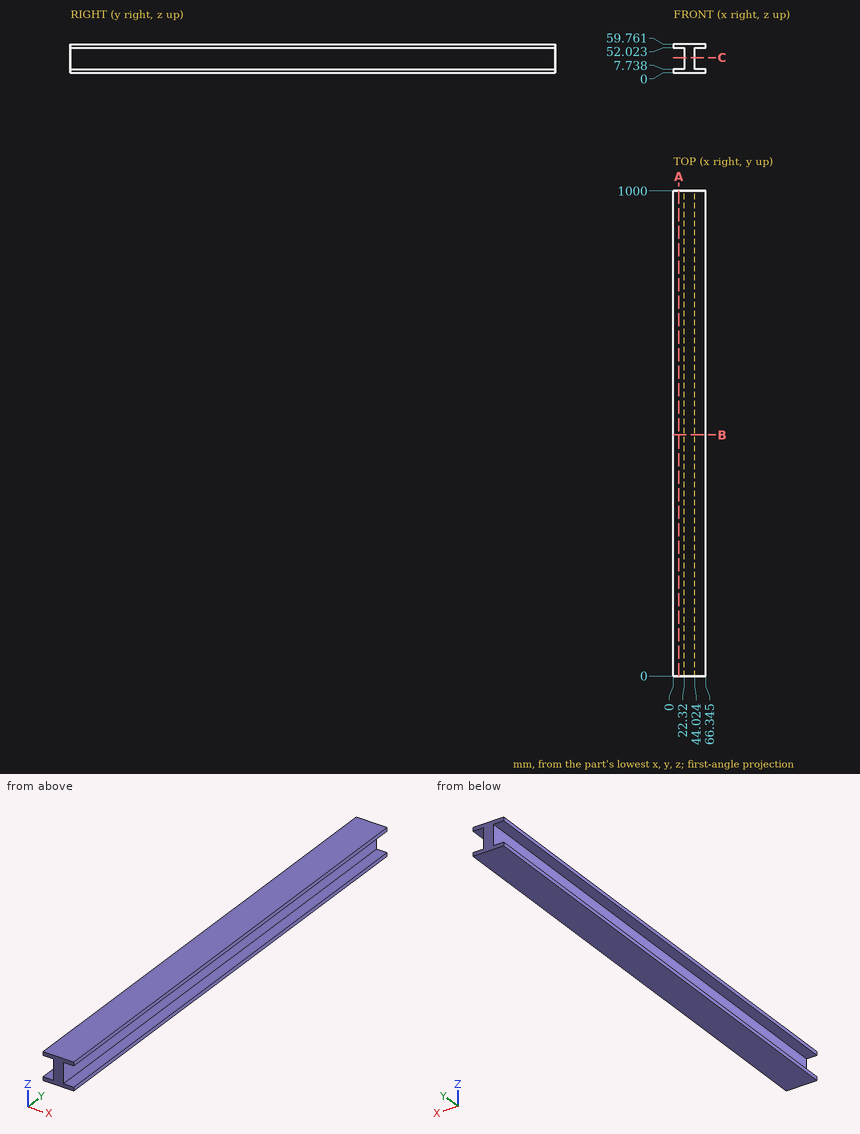
Geometry: see drawing. Coordinates: mm, zero at the bounding-box minimum. Round coordinates to 2 decimals unless told otherwise and drop trailing zeros. Loops run counter-clockwise (first coordinate to the right, second up) from the corner with the lowest first, then second, coordinate; pieces in that order, holes last. Notation, with made-up numbers: M 25,-21 L 75,-21 A5 ccw 75,-14 Z; hole C 79,88 d2. An arc over 180 degrees is marked long. Use a Markdown table: item, result. Add a question column.
1. Cut plane A-A, the plane x = 11.5. Output: boundary loops of the cut face in (y, z).
2. Contact query for flat-ended pins moving along their axis: pin 1 (8 mm diameter, centred on y = 384, z = 34, fed in from +X); pin 2 (8 mm diameter, centred on y = 864, z = 43, fed in from -X). Output: stop coordinate, or through.
3. Cut plane C-C, the plane z = 31.5. Output: boundary loops of the cut face in (x, y) (1 decimal).
4. Ray query, line 1 along Z through (x, y) = (46, 421); line 2 along X through (y, z) = (181.5, 21) (1 decimal). Return the intervals inside material, ascending. Write a range as [from, to].
5. Cut plane B-B, the plane y = 497. Output: boundary loops of the cut face in (x, z) (1 decimal).
Solution:
| question | item | result |
|---|---|---|
| 1 | outline | M 0,0 L 1000,0 L 1000,7.74 L 0,7.74 Z; M 0,52.02 L 1000,52.02 L 1000,59.76 L 0,59.76 Z |
| 2 | pin 1 | stops at x = 44.02 |
| 2 | pin 2 | stops at x = 22.32 |
| 3 | outline | M 22.3,0 L 44,0 L 44,1000 L 22.3,1000 Z |
| 4 | line 1 | z = [0, 7.74], [52.02, 59.76] |
| 4 | line 2 | x = [22.3, 44] |
| 5 | outline | M 0,0 L 66.3,0 L 66.3,7.7 L 44,7.7 L 44,52 L 66.3,52 L 66.3,59.8 L 0,59.8 L 0,52 L 22.3,52 L 22.3,7.7 L 0,7.7 Z |
